For this review, take the finished solid that the model builds, in its own axes (mm). Face numbers are marked on the shaded views. Coordinates: 2 decimals unless noted, no trailing zeros. Loops run counter-clockwise (first coordinate to the right, second up) from the corner with the lowest first, then second, coordinate; pieces in that order, holes last. Notation, with made-up numbers: (4, 74) - (26, 74) arc R18 cw to (26, 80) - close; hole circle Ø6 at (-20, 73.5). An arc over 180 degrees is marked (long way). One line per item, written item: value. Start each with the question number.
1. Take a section at A-A, the plane z = -1.45. Count the separate pieces of the cut face and the enclosed holes in it, and give its area (3 significant figures).
2. Take a section at D-D, the plane y = 10. State the section outline as (x, z) points.
3. Take a section at C-C, the plane x = 11. State the section outline as (y, z) points, and give its area (3 significant figures).
4. Insertion check: pin 1 (1 mm diameter, centred on y = -0.5, z = -1.5, fed in from +X); pin 2 (10 mm diameter, centred on x = 30.5, y = -2.5, fed in from -Z); pin 3 (1 mm diameter, centred on x = 18.5, z = -2, fed in from +Y). Each pin has a flat end and moves straight along its axis. Give the tip position at first contact, or say it passes through.
5. The part is to be moulded in two halves that separate along X. For the marked faces 1, 2, 3 and 4, say which applies: released by +X, released by -X, zero draft, split by the parting line, or undercut.
6. Take a section at B-B, the plane y = 0. State the section outline as (x, z) points.
7. To check wall thickness, follow line 1 (X direction, y = 0.25, z = -0.4); line 2 (X direction, y = -0.5, z = -2.55); line 3 (Y direction, x = 6.5, z = -1.55). State the ranges of each line that lie inside material, in increasing order. Write a range as from..to.
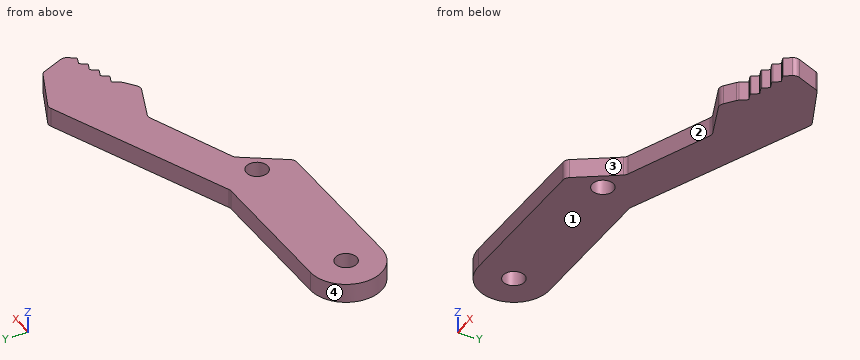
```python
from build123d import *

# Parameters (mm, degrees)
SKETCH1_R           = 1.5
BOSS_EXTRUDE1_DEPTH = 2.7
FILLET1_R           = 0.15
FILLET2_R           = 1
FILLET3_R           = 1
FILLET4_R           = 1


with BuildPart() as part:
    # Sketch1 → Boss-Extrude1 (new body)
    with BuildSketch(Plane.XY):
        with BuildLine():
            Line((0, 5), (19.85, 5))
            Line((19.85, 5), (45.99619398, 15.75))
            Line((45.99619398, 15.75), (52.557536486, 12.761206845))
            Line((52.557536486, 12.761206845), (53.907471601, 9.477889135))
            ThreePointArc((53.907471601, 9.477889135), (53.977314115, 8.995006796), (53.810360044, 8.536553233))
            Line((53.810360044, 8.536553233), (53.148294507, 7.559788561))
            Line((53.148294507, 7.559788561), (52.056234711, 8.006784537))
            Line((52.056234711, 8.006784537), (51.394169174, 7.030019865))
            Line((51.394169174, 7.030019865), (50.302109378, 7.477015841))
            Line((50.302109378, 7.477015841), (49.640043841, 6.500251169))
            Line((49.640043841, 6.500251169), (48.547984045, 6.947247144))
            Line((48.547984045, 6.947247144), (47.885918508, 5.970482472))
            Line((47.885918508, 5.970482472), (46.793858712, 6.417478448))
            Line((46.793858712, 6.417478448), (46.131793175, 5.440713776))
            ThreePointArc((46.131793175, 5.440713776), (46.03170075, 5.315863389), (45.912975416, 5.208576821))
            Line((45.912975416, 5.208576821), (44.507662892, 4.129714813))
            ThreePointArc((44.507662892, 4.129714813), (44.031433487, 3.93177062), (43.519903831, 3.997449854))
            Line((43.519903831, 3.997449854), (38.212047423, 6.170032768))
            Line((38.212047423, 6.170032768), (25.644379319, 1.158584034))
            Line((25.644379319, 1.158584034), (21.47, -5))
            Line((21.47, -5), (0, -5))
            ThreePointArc((0, -5), (-5, 0), (0, 5))
        make_face()
        Circle(SKETCH1_R, mode=Mode.SUBTRACT)
        with Locations((22, 0)):
            Circle(SKETCH1_R, mode=Mode.SUBTRACT)
    extrude(amount=-BOSS_EXTRUDE1_DEPTH)

    # Fillet1
    fillet1_edges = [part.edges().sort_by_distance(p)[0] for p in [
        (53.148294507, 7.559788561, -1.35),
        (51.394169174, 7.030019865, -1.35),
        (49.640043841, 6.500251169, -1.35),
        (47.885918508, 5.970482472, -1.35),
    ]]
    fillet(fillet1_edges, radius=FILLET1_R)

    # Fillet2
    fillet2_edges = [part.edges().sort_by_distance(p)[0] for p in [
        (21.47, -5, -1.35),
        (45.99619398, 15.75, -1.35),
        (52.557536486, 12.761206845, -1.35),
    ]]
    fillet(fillet2_edges, radius=FILLET2_R)

    # Fillet3
    fillet3_edges = [part.edges().sort_by_distance(p)[0] for p in [
        (38.212047423, 6.170032768, -1.35),
        (25.644379319, 1.158584034, -1.35),
    ]]
    fillet(fillet3_edges, radius=FILLET3_R)

    # Fillet4
    fillet4_edges = [part.edges().sort_by_distance(p)[0] for p in [
        (19.85, 5, -1.35),
    ]]
    fillet(fillet4_edges, radius=FILLET4_R)


solid = part.part
```
Solutions:
1. separate pieces: 1
1. enclosed holes: 2
1. area: 480 mm2
2. outline: (32.01, -2.7) - (53.69, -2.7) - (53.69, 0) - (32.01, 0) - close
3. outline: (-5, -2.7) - (5, -2.7) - (5, 0) - (-5, 0) - close
3. area: 27.0 mm2
4. pin 1: x = 24.86
4. pin 2: through
4. pin 3: y = 5
5. face 1: zero draft
5. face 2: undercut
5. face 3: released by +X
5. face 4: released by -X
6. outline: (-5, -2.7) - (-1.5, -2.7) - (-1.5, 0) - (-5, 0) - close; (1.5, -2.7) - (20.5, -2.7) - (20.5, 0) - (1.5, 0) - close; (23.5, -2.7) - (24.86, -2.7) - (24.86, 0) - (23.5, 0) - close
7. line 1: -4.99..-1.48, 1.48..20.52, 23.48..25.03
7. line 2: -4.97..-1.41, 1.41..20.59, 23.41..24.52
7. line 3: -5..5
